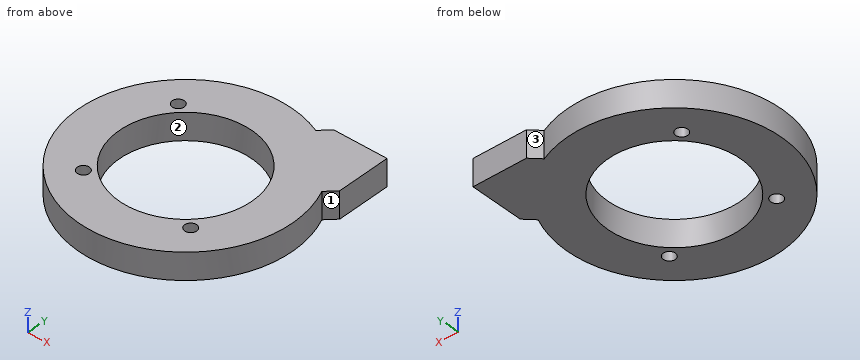
```python
from build123d import *

# Parameters (mm, degrees)
SKETCH1_R           = 15.748
BOSS_EXTRUDE1_DEPTH = 6.35
SKETCH2_R           = 1.4224
CUT_EXTRUDE2_DEPTH  = 6.35


with BuildPart() as part:
    # Sketch1 → Boss-Extrude1 (new body)
    with BuildSketch(Plane.XY):
        with BuildLine():
            Line((23.150520825, 10.450520825), (25.4, 12.7))
            Line((25.4, 12.7), (25.4, 25.4))
            Line((25.4, 25.4), (12.7, 25.4))
            Line((12.7, 25.4), (10.450520825, 23.150520825))
            ThreePointArc((10.450520825, 23.150520825), (-17.960512242, -17.960512242), (23.150520825, 10.450520825))
        make_face()
        Circle(SKETCH1_R, mode=Mode.SUBTRACT)
    extrude(amount=BOSS_EXTRUDE1_DEPTH)

    # Sketch2 → Cut-Extrude2 (cut)
    with BuildSketch(Plane.XY.offset(6.35)):
        with Locations((12.76910233, -13.056515019)):
            Circle(SKETCH2_R)
        with Locations((-13.056515019, 12.76910233)):
            Circle(SKETCH2_R)
        with Locations((-12.76910233, -13.056515019)):
            Circle(SKETCH2_R)
    extrude(amount=-CUT_EXTRUDE2_DEPTH, mode=Mode.SUBTRACT)


solid = part.part
```
The listing builds one solid part. Answer for the finished solid, in the listing's coordinates (mm). Face numbers are marked on the shaded views. A direction names the side the tool comes from. Round coordinates to 2 decimals unless told otherwise and drop trailing zeros. Loops run counter-clockwise (first coordinate to the right, second up) from the corner with the lowest first, then second, coordinate; pieces in that order, holes last. Notation, with made-up numbers: (69.25, 30.25) - (81.25, 30.25) arc R28 ccw to (81.25, 60.25) - close; hole circle Ø5 at (-5, 0). An arc over 180 degrees is marked (long way). Return JSON: item names as keys, results as strings. Group by question number.
1. The part is cut by section B-B on x = 2. Determine the outline of the cut face in (y, z).
2. Which of the six approach directions +Z, -Z, +X, -X, +Y, -Y give full straight-line access (tool end or side, diameter ignored) to the marked faces 1, 2 and 3?
3. The part is cut by section A-A on y = 0. Determine the outline of the cut face in (x, z), then the cut area to 3 significant figures.
4. The part is cut by section C-C on z = 5.5. Determine the outline of the cut face in (x, y).
5. Each of these flat-tipped pins is pushed along its axis until it touches: P1, Ø6, axis at x = -11, y = -10, coming from the +Z side; P2, Ø3, axis at x = 2.5, y = 13.5, coming from the +Z side; P3, Ø3, axis at y = -16, z = 2, coming from the +X side. Where does it stop, or does it pass through?
6. The part is cut by section D-D on x = -17.5. Determine the outline of the cut face in (y, z).
7. Consider probe 1 along Y at (x, z) = (13.5, 4.25); probe 2 along Y at (x, z) = (0, 3.25); probe 3 along X at (y, z) = (-12, 2.75). Determine where each line is inside the solid, lowest interval first.
Resolved:
{
 "1": {"outline": "(-25.32, 0) - (-15.62, 0) - (-15.62, 6.35) - (-25.32, 6.35) - close; (15.62, 0) - (25.32, 0) - (25.32, 6.35) - (15.62, 6.35) - close"},
 "2": {"face 1": "+Z, -Z, +X", "face 2": "+Z, -Z", "face 3": "+Z, -Z, +Y"},
 "3": {"outline": "(-25.4, 0) - (-15.75, 0) - (-15.75, 6.35) - (-25.4, 6.35) - close; (15.75, 0) - (25.4, 0) - (25.4, 6.35) - (15.75, 6.35) - close", "area": "123 mm²"},
 "4": {"outline": "(10.45, 23.15) arc R25.4 ccw (long way) to (23.15, 10.45) - (25.4, 12.7) - (25.4, 25.4) - (12.7, 25.4) - close; hole circle Ø31.5 at (0, 0); hole circle Ø2.84 at (-13.06, 12.77); hole circle Ø2.84 at (-12.77, -13.06); hole circle Ø2.84 at (12.77, -13.06)"},
 "5": {"P1": "stops at z = 6.35", "P2": "passes through", "P3": "stops at x = 20.85"},
 "6": {"outline": "(-18.41, 0) - (18.41, 0) - (18.41, 6.35) - (-18.41, 6.35) - close"},
 "7": {"probe 1": "y = -21.52 to -14.28, -11.84 to -8.11, 8.11 to 25.4", "probe 2": "y = -25.4 to -15.75, 15.75 to 25.4", "probe 3": "x = -22.39 to -13.72, -11.82 to -10.2, 10.2 to 11.82, 13.72 to 22.39"}
}
